from build123d import *

# Parameters (mm, degrees)
BOSS_EXTRUDE3_DEPTH                    = 8
SKETCH8_R                              = 6.884606738
CUT_EXTRUDE3_DEPTH                     = 88
F_39_0_0995_DIAMETER_HOLE1_D           = 2.5273
F_39_0_0995_DIAMETER_HOLE1_ON_FACE_2_D = 2.5273


with BuildPart() as part:
    # Sketch6 → Boss-Extrude3 (new body)
    with BuildSketch(Plane(origin=(0, 0, 0), x_dir=(1, 0, 0), z_dir=(0, 1, 0))):
        Polygon((-16.836914056, 5.783353512), (13.163085944, 5.783353512), (33.163085944, -49.166194877), (-36.836914056, -49.166194877), align=None)
    extrude(amount=BOSS_EXTRUDE3_DEPTH)

    # Sketch8 → Cut-Extrude3 (cut)
    with BuildSketch(Plane.XY.offset(49.166194877)):
        with Locations((-1.836914056, 0)):
            Circle(SKETCH8_R)
    extrude(amount=-CUT_EXTRUDE3_DEPTH, mode=Mode.SUBTRACT)

    # #39 (0.0995) Diameter Hole1 (through all)
    with Locations(Plane(origin=(17.988085944, 8, 24.13287332), x_dir=(0, 0, 1), z_dir=(0, 1, 0))):
        with Locations((0, 0), (18.916226832, 4.825), (18.916226832, -44.475), (-18.916226832, -34.825), (-18.916226832, -4.825), (0, -39.65)):
            Hole(F_39_0_0995_DIAMETER_HOLE1_D / 2)

    # #39 (0.0995) Diameter Hole1 on face 2 (through all)
    with Locations(Plane(origin=(-16.836914056, 0, 5.216646488), x_dir=(0, 0, -1), z_dir=(0, -1, 0))):
        with Locations((0, 0), (0, 30), (-37.832453664, 39.65), (-37.832453664, -9.65)):
            Hole(F_39_0_0995_DIAMETER_HOLE1_ON_FACE_2_D / 2)


solid = part.part
Verification items for the finished model (mm, model axes). Give positions to 0.01 mm unless a question says otherwise; leave off trailing zeros. Write each loop counter-clockwise with the first axis right and the second up, starting at its lowest first coordinate (ties: lowest second). Pieces come first, ordered by that corner, then holes. Notation, with made-up numbers: M -33.5,-8 L 19.5,-8 A18 ccw 19.5,20 Z; hole C 61.5,29 d8. An arc over 180 degrees is marked long. Put each result on its own line as item: value. Start each with the question number.
1. Draft check along X on faces 1 (the face through (22.33, 3.94, 41.88)), 2 (the face through (-1, 8, 27)), 3 (the face through (-26.98, 3.94, 22.08)). Enter one of: +X half, -X half, draft (parallel to the pull), parting line (faces both ways), or undercut.
2. Section check D-D (x = 27.5). Record the cut outline in (y, z), and give its area (3 significant figures).
3. Section check C-C (x = -29.5). Record the cut outline in (y, z).
4. Section check B-B (z = 28.5). Record the cut outline in (x, y).
5. Go/stop test with a flat-tipped pin: pin 1 Ø1.5 at (y, z) = (3.5, 3) entering from -X. Record where the tip stops, or that it passes through.
6. Scan lines: line 1 along X through (y, z) = (4.75, 4.5); line 2 along X through (y, z) = (2.5, 25); line 3 along X through (y, z) = (1, 41). Record each from-to range of solid material in increasing order. Write a range as [from, to].
7. Section check A-A (y = 3.25). Record the cut outline in (x, z).
Answer list:
1. face 1: undercut
1. face 2: draft
1. face 3: -X half
2. outline: M 0,33.61 L 8,33.61 L 8,49.17 L 0,49.17 Z
2. area: 124 mm2
3. outline: M 0,29.01 L 8,29.01 L 8,49.17 L 0,49.17 Z
4. outline: M -29.32,0 L -8.72,0 A6.88 cw 5.05,0 L 25.64,0 L 25.64,8 L -29.32,8 Z
5. pin 1: x = -20.31
6. line 1: [-20.58, -17.88], [-15.8, -6.82], [3.15, 12.12], [14.2, 16.91]
6. line 2: [-28.04, -22.58], [-20.74, -8.25], [4.58, 17.07], [18.91, 24.37]
6. line 3: [-33.86, -8.65], [4.97, 30.19]
7. outline: M -36.84,49.17 L -16.84,-5.78 L -7.91,-5.78 L -7.91,49.17 Z; M 4.23,-5.78 L 13.16,-5.78 L 33.16,49.17 L 4.23,49.17 Z; hole C -26.49,43.05 d2.53; hole C -21.66,24.13 d2.53; hole C -16.84,5.22 d2.53; hole C 13.16,5.22 d2.53; hole C 17.99,24.13 d2.53; hole C 22.81,43.05 d2.53
